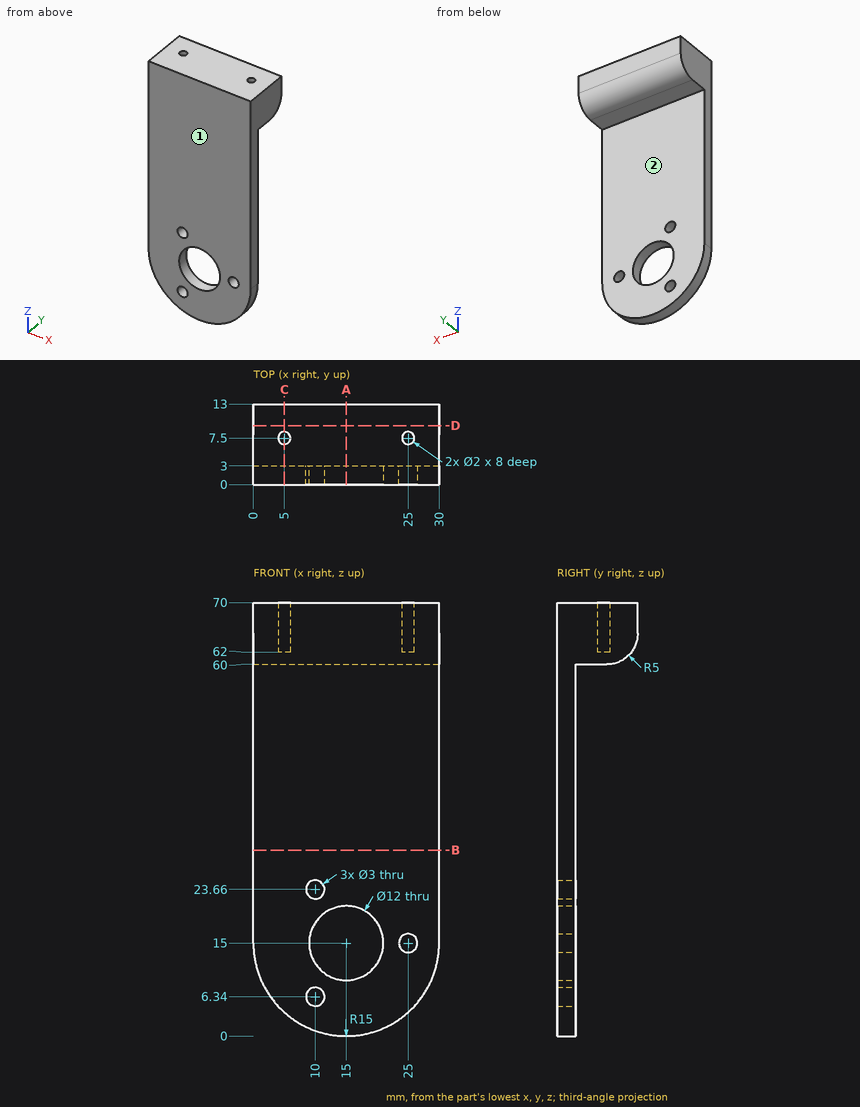
Source: three-view drawing plus pictorial views. Frame: mm from the lowest corner of the part. A direction names the side the tool comes from. Coordinates: 2 decimals unless noted, no trailing zeros. Order: outer loops, then holes, each group sorted by start corner. A loop starts at its lowest first (then second) coordinate and runs counter-clockwise, first axis right, second up. Notation, with made-up numbers: M -37.75,63.25 L -4.75,63.25 A18 ccw -4.75,79.25 Z; hole C 87.5,44.5 d4. An arc over 180 degrees is marked long. One line per question, with ' | ' between items.
Item 1: Section B-B (z = 30). Output: boundary loops of the cut face in (x, y).
Geometry results:
outline: M 0,0 L 30,0 L 30,3 L 0,3 Z
Item 2: Reachability of the marked faces 1 and 2 from +Z, -Z, +X, -X, +Y, -Y: full face, straight path, thin tool, end or side. Return the list, or none.
Geometry results:
face 1: +Z, -Z, +X, -X, -Y | face 2: -Z, +X, -X, +Y
Item 3: Section D-D (y = 9.5). Output: boundary loops of the cut face in (x, z), then the cut area to 3 significant figures.
Geometry results:
outline: M 0,60.23 L 30,60.23 L 30,70 L 0,70 Z | area: 293 mm^2
Item 4: Section C-C (x = 5). Output: boundary loops of the cut face in (y, z).
Geometry results:
outline: M 0,3.82 L 3,3.82 L 3,60 L 8,60 A5 ccw 13,65 L 13,70 L 8.5,70 L 8.5,62 L 6.5,62 L 6.5,70 L 0,70 Z
Item 5: Section A-A (x = 15). Output: boundary loops of the cut face in (y, z).
Geometry results:
outline: M 0,0 L 3,0 L 3,9 L 0,9 Z; M 0,21 L 3,21 L 3,60 L 8,60 A5 ccw 13,65 L 13,70 L 0,70 Z
Item 6: Ray query, line 1 along Y through (x, z) = (25, 66.5); line 2 along Z through (x, y) = (10, 1) (1 decimal); line 3 along Z through (x, y) = (15, 1.6). Return the intervals inside material, ascending.
Geometry results:
line 1: y = 0 to 6.5, 8.5 to 13 | line 2: z = 0.9 to 4.8, 7.8 to 11.7, 18.3 to 22.2, 25.2 to 70 | line 3: z = 0 to 9, 21 to 70
Item 7: Pin query (flat end, axial travel): pin 1 (3 mm diameter, centred on x = 13, y = 7, fed in from -Z); pin 2 (5.5 mm diameter, centred on x = 16.5, y = 5.5, fed in from -Z); pin 3 (2 mm diameter, centred on x = 5, y = 7, fed in from +Z); pin 4 (11 mm diameter, centred on x = 15, z = 15, fed in from +Y). Return the tip coordinate at first contact, or that it passes through.
Geometry results:
pin 1: stops at z = 60 | pin 2: stops at z = 0 | pin 3: stops at z = 70 | pin 4: passes through
